Source: CAD feature listing. Evaluate the final solid. Frame: model axes, mm. Round coordinates to 2 decimals unless told otherwise and drop trailing zeros. Loops run counter-clockwise (first coordinate to the right, second up) from the corner with the lowest first, then second, coordinate; pieces in that order, holes last.
Item 1: Section query D-D on z = 101.25. Return loops of the section in (x, y), then the cut area to 3 significant figures.
Item 2: Section query B-B on y = 0.35. Return loops of the section in (x, z), then the cut area to 3 significant figures.
Item 3: First-contact query: P1, Ø2.5, axis at x = 19.41, z = 92.68, coming from the -Y side; P2, Ø1.8, axis at x = 4.41, z = 104.43, coming from the -Y side. Flat tips, straight axial feed; report the tip coordinate or a pass-through.
Item 4: Ray query, L1, parallel to Z at x = 4.5, y = 0.6; L2, parallel to Z at x = 19.5, y = 0.9; L3, parallel to X at y = 0.8, z = 80.75. Return the intervals inside material, ascending.
Item 5: Pull-direction query (Z, two-part tool) for faces 1 (the cylindrical face through (4.457, 0.507, 79.935)), 2 (the cylindrical face through (20.404, 0.507, 92.554)), 3 (the flat face through (-13.587, 0.5, 92.8)), 4 (the flat face through (5.2, 0.5, 78.684)); classes: released by +Z, released by -Z, zero draft, split by the parting line, or undercut.
Item 6: Section query C-C on x = 23. Return loops of the section in (y, z), then the cut area to 3 significant figures.
Item 7: Section query A-A on z = 81.25. Return loops of the section in (x, y).
```python
from build123d import *

# Parameters (mm, degrees)
BOSS_EXTRUDE1_DEPTH = 1
SKETCH2_R           = 1
CUT_EXTRUDE1_DEPTH  = 1
SKETCH4_R           = 1
CUT_EXTRUDE2_DEPTH  = 1


with BuildPart() as part:
    # Sketch1 → Boss-Extrude1 (new body)
    with BuildSketch(Plane(origin=(0, 0, 0), x_dir=(1, 0, 0), z_dir=(0, 1, 0))):
        Polygon((-13.58704372, -102.683820402), (-13.58704372, -82.683820402), (-9.58704372, -78.683820402), (20.41295628, -78.683820402), (27.41295628, -85.683820402), (27.41295628, -99.683820402), (20.41295628, -106.683820402), (-9.58704372, -106.683820402), align=None)
    extrude(amount=BOSS_EXTRUDE1_DEPTH)

    # Sketch2 → Cut-Extrude1 (cut)
    with BuildSketch(Plane(origin=(0, 1, 0), x_dir=(1, 0, 0), z_dir=(0, 1, 0))):
        with Locations(Location((19.41295628, -92.683820402, 0), (0, 0, 270))):
            Circle(SKETCH2_R)
    extrude(amount=-CUT_EXTRUDE1_DEPTH, mode=Mode.SUBTRACT)

    # Sketch4 → Cut-Extrude2 (cut)
    with BuildSketch(Plane(origin=(0, 1, 0), x_dir=(1, 0, 0), z_dir=(0, 1, 0))):
        with Locations(Location((4.41295628, -104.433820402, 0), (0, 0, 270))):
            Circle(SKETCH4_R)
        with Locations(Location((4.41295628, -80.933820402, 0), (0, 0, 270))):
            Circle(SKETCH4_R)
    extrude(amount=-CUT_EXTRUDE2_DEPTH, mode=Mode.SUBTRACT)


solid = part.part
```
Data:
1. outline: (-13.59, 0) - (25.85, 0) - (25.85, 1) - (-13.59, 1) - close
1. area: 39.4 mm2
2. outline: (-13.59, 82.68) - (-9.59, 78.68) - (20.41, 78.68) - (27.41, 85.68) - (27.41, 99.68) - (20.41, 106.68) - (-9.59, 106.68) - (-13.59, 102.68) - close; hole circle Ø2 at (4.41, 80.93); hole circle Ø2 at (4.41, 104.43); hole circle Ø2 at (19.41, 92.68)
2. area: 1,070 mm2
3. P1: stops at y = 0
3. P2: passes through
4. L1: z = 78.68 to 79.94, 81.93 to 103.44, 105.43 to 106.68
4. L2: z = 78.68 to 91.69, 93.68 to 106.68
4. L3: x = -11.65 to 3.43, 5.4 to 22.48
5. face 1: undercut
5. face 2: undercut
5. face 3: zero draft
5. face 4: released by -Z
6. outline: (0, 81.27) - (1, 81.27) - (1, 104.1) - (0, 104.1) - close
6. area: 22.8 mm2
7. outline: (-12.15, 0) - (3.46, 0) - (3.46, 1) - (-12.15, 1) - close; (5.36, 0) - (22.98, 0) - (22.98, 1) - (5.36, 1) - close
